from build123d import *

# Parameters (mm, degrees)
CROQUIS1_W              = 42
CROQUIS1_H              = 65
CROQUIS1_R              = 2.05
SALIENTE_EXTRUIR1_DEPTH = 4
CROQUIS5_R              = 5
CORTAR_EXTRUIR2_DEPTH   = 5
CROQUIS6_W              = 42
CROQUIS6_H              = 7.7
SALIENTE_EXTRUIR2_DEPTH = 4
CHAFL_N1_SIZE           = 4.1


with BuildPart() as part:
    # Croquis1 → Saliente-Extruir1 (new body)
    with BuildSketch(Plane.XY):
        with Locations((21, 32.5)):
            Rectangle(CROQUIS1_W, CROQUIS1_H)
        with Locations((11, 56.8)):
            Circle(CROQUIS1_R, mode=Mode.SUBTRACT)
        with Locations((31, 56.8)):
            Circle(CROQUIS1_R, mode=Mode.SUBTRACT)
    extrude(amount=SALIENTE_EXTRUIR1_DEPTH)

    # Croquis5 → Cortar-Extruir2 (cut, through all)
    with BuildSketch(Plane.XY.offset(4)):
        with Locations((21, 21.08)):
            Circle(CROQUIS5_R)
    extrude(amount=-CORTAR_EXTRUIR2_DEPTH, mode=Mode.SUBTRACT)

    # Croquis6 → Saliente-Extruir2 (add, through all)
    with BuildSketch(Plane.XY.offset(4)):
        with Locations((21, -3.85)):
            Rectangle(CROQUIS6_W, CROQUIS6_H)
    extrude(amount=-SALIENTE_EXTRUIR2_DEPTH)

    # Chaflán1
    chafl_n1_edges = [part.edges().sort_by_distance(p)[0] for p in [
        (0, -7.7, 2),
        (42, -7.7, 2),
    ]]
    chamfer(chafl_n1_edges, length=CHAFL_N1_SIZE)


solid = part.part
For this review, take the finished solid that the model builds, in its own axes (mm). Round coordinates to 2 decimals unless told otherwise and drop trailing zeros. Write each loop counter-clockwise with the first axis right and the second up, starting at its lowest first coordinate (ties: lowest second). Pieces come first, ordered by that corner, then holes. Notation, with made-up numbers: (24.25, -34) - (41.25, -34) arc R33 ccw to (41.25, -6) - close; hole circle Ø8 at (-16.5, 43.5). An arc over 180 degrees is marked (long way). Use a Markdown table: item, result.
Q1. We need section D-D (y = 56.8). Give the boundary of the cut face in (x, z).
Derived:
| item | result |
|---|---|
| outline | (0, 0) - (8.95, 0) - (8.95, 4) - (0, 4) - close; (13.05, 0) - (28.95, 0) - (28.95, 4) - (13.05, 4) - close; (33.05, 0) - (42, 0) - (42, 4) - (33.05, 4) - close |
Q2. Wall thickness on line 1 along Y through (x, z) = (31, 1.85); line 2 along Y through (x, z) = (21, 2.5); line 3 along X through (y, z) = (17.5, 2.1): over which ranges is each line inside the solid? List them lowest first.
Derived:
| item | result |
|---|---|
| line 1 | y = -7.7 to 54.75, 58.85 to 65 |
| line 2 | y = -7.7 to 16.08, 26.08 to 65 |
| line 3 | x = 0 to 17.51, 24.49 to 42 |
Q3. We need section A-A (x = 21). Give the boundary of the cut face in (y, z).
Derived:
| item | result |
|---|---|
| outline | (-7.7, 0) - (16.08, 0) - (16.08, 4) - (-7.7, 4) - close; (26.08, 0) - (65, 0) - (65, 4) - (26.08, 4) - close |
Q4. We need section B-B (y = 21.08). Give the boundary of the cut face in (x, z), plus the area to 3 significant figures.
Derived:
| item | result |
|---|---|
| outline | (0, 0) - (16, 0) - (16, 4) - (0, 4) - close; (26, 0) - (42, 0) - (42, 4) - (26, 4) - close |
| area | 128 mm2 |
Q5. The part is to be moulded in two halves that separate along Y. For faces 1 (the cylindrical face through (30.556, 54.799, 1.972)), 2 (the flat face through (21, 65, 2)), 3 (the flat face through (39.9, -5.7, 2)), say which applies: pulls with the +Y half, pulls with the -Y half, needs draft (parallel to the pull), parting line crosses it, or undercut.
Derived:
| item | result |
|---|---|
| face 1 | undercut |
| face 2 | pulls with the +Y half |
| face 3 | pulls with the -Y half |
Q6. We need section C-C (z = 0.65). Give the boundary of the cut face in (x, y), plus the area to 3 significant figures.
Derived:
| item | result |
|---|---|
| outline | (0, -3.6) - (4.1, -7.7) - (37.9, -7.7) - (42, -3.6) - (42, 65) - (0, 65) - close; hole circle Ø4.1 at (11, 56.8); hole circle Ø10 at (21, 21.08); hole circle Ø4.1 at (31, 56.8) |
| area | 2,930 mm2 |
